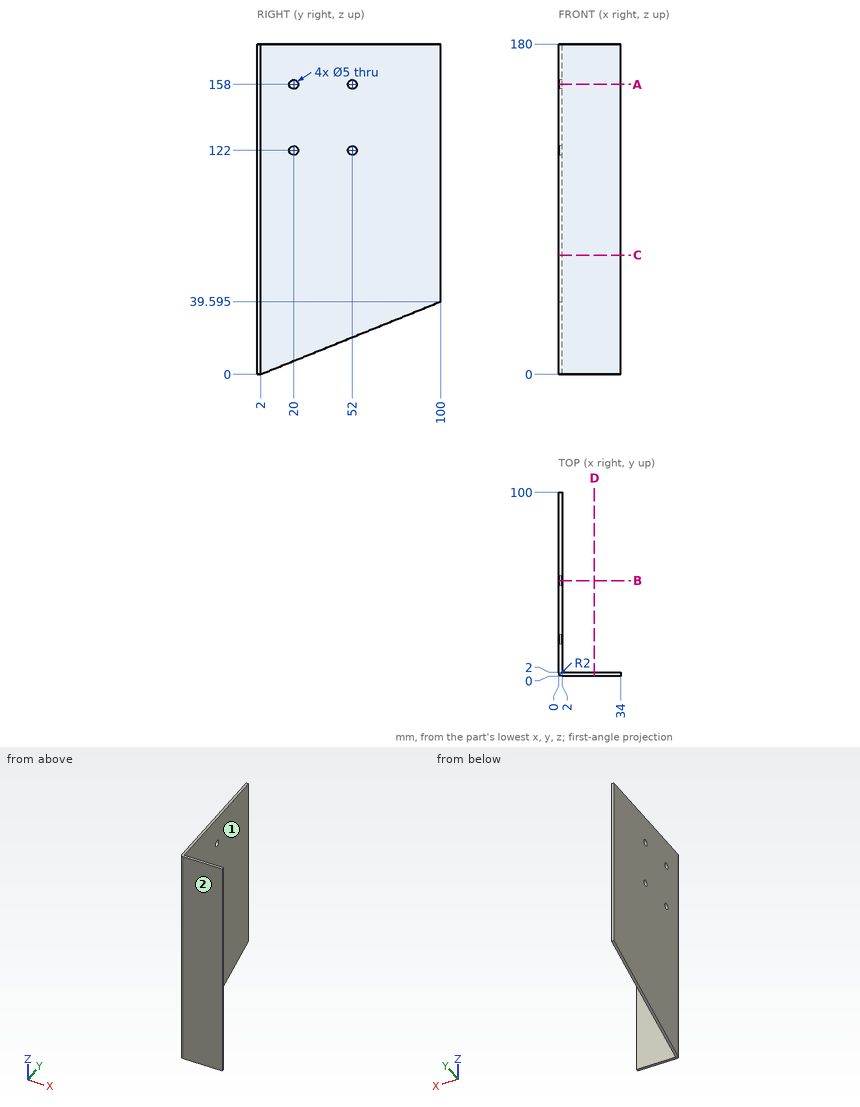
Design review of the part shown in the three views and the two pictorial views. Dimensions are in mm from the part's minimum x, y and z. A direction names the side the tool comes from. Round coordinates to 2 decimals unless told otherwise and drop trailing zeros. Order: outer loops, then holes, each group sorted by start corner. A loop starts at its lowest first (then second) coordinate and runs counter-clockwise, first axis right, second up. Notation, with made-up numbers: (9, 38.25) -> (65, 38.25) arc R38 cw to (65, 76.25) -> close; hole circle Ø2 at (74.5, -36). An arc over 180 degrees is marked (long way). Write item = value, one per line. Start each with the question number.
1) To check wall thickness, follow line 1 (X direction, y = 11, z = 103); line 2 (Y direction, x = 0.65, z = 122) (1 decimal). State the ranges of each line that lie inside material, in increasing order. Write a range as from..to.
2) Take a section at D-D on x = 19.5. State the section outline as (y, z) points, plus the area to 3 significant figures.
3) Take a section at B-B on y = 52. State the section outline as (x, z) points.
4) Insertion check: pin 1 (5 mm diameter, centred on x = 15.5, z = 104.5, fed in from +Y); pin 2 (1 mm diameter, centred on y = 62, z = 120, fed in from +X); pin 3 (3 mm diameter, centred on y = 52, z = 122, fed in from -X). Each pin has a flat end and moves straight along its axis. Give the tip position at first contact, or say it passes through.
5) Tool access review of the marked faces 1 and 2: name each direction out of +Z, -Z, +X, -X, +Y, -Y from which nothing blocks a thin tool from reaching the whole face with its end or side.
6) Take a section at A-A on z = 158. State the section outline as (x, y) points.
7) Take a section at C-C on z = 65. State the section outline as (x, y) points.
Verdict:
q1.line_1 = 0..2
q1.line_2 = 0.5..17.5, 22.5..49.5, 54.5..100
q2.outline = (0, 0) -> (2, 0) -> (2, 180) -> (0, 180) -> close
q2.area = 360 mm2
q3.outline = (0, 20.2) -> (2, 20.2) -> (2, 119.5) -> (0, 119.5) -> close; (0, 124.5) -> (2, 124.5) -> (2, 155.5) -> (0, 155.5) -> close; (0, 160.5) -> (2, 160.5) -> (2, 180) -> (0, 180) -> close
q4.pin_1 = 2
q4.pin_2 = 2
q4.pin_3 = through
q5.face_1 = +Z, -Z, +X, +Y
q5.face_2 = +Z, -Z, +X, -X, -Y
q6.outline = (0, 2) arc R2 ccw to (2, 0) -> (34, 0) -> (34, 2) -> (2, 2) -> (2, 17.5) -> (0, 17.5) -> close; (0, 22.5) -> (2, 22.5) -> (2, 49.5) -> (0, 49.5) -> close; (0, 54.5) -> (2, 54.5) -> (2, 100) -> (0, 100) -> close
q7.outline = (0, 2) arc R2 ccw to (2, 0) -> (34, 0) -> (34, 2) -> (2, 2) -> (2, 100) -> (0, 100) -> close
